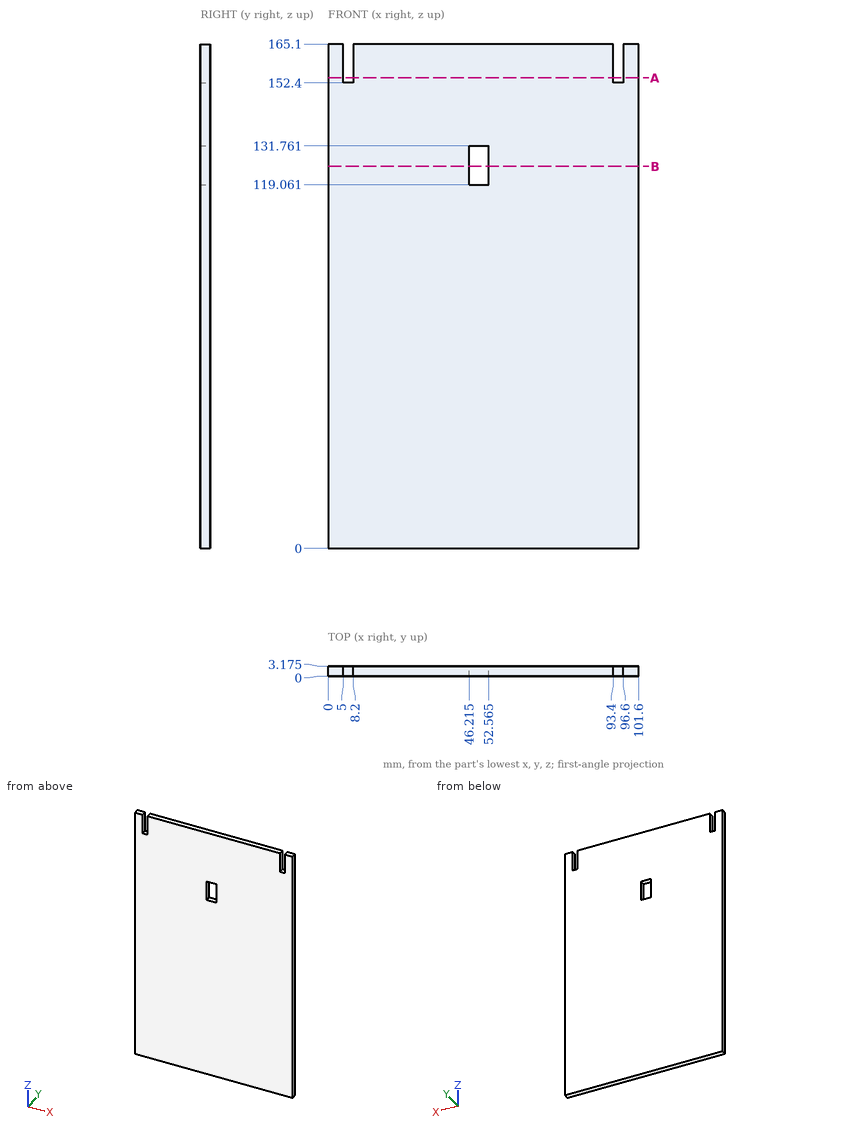
Geometry check sheet. Reference: drawing and pictorial views, mm from the part's lowest x, y, z. Give positions to 0.01 mm unless a question says otherwise; leave off trailing zeros. Loops run counter-clockwise (first coordinate to the right, second up) from the corner with the lowest first, then second, coordinate; pieces in that order, holes last. Notation, with made-up numbers: (-8.5, 63.5) - (34.5, 63.5) arc R29 ccw to (34.5, 102.5) - close; hole circle Ø6 at (65, -38.75). An arc over 180 degrees is marked (long way). Use CSV: the item, a comma, the result in double quotes. Start each with the question number.
Q1. Section check B-B, the plane z = 125. Record the cut outline in (x, y) (1 decimal).
Q2. Go/stop test with a flat-tipped pin: pin 1 Ø1.6 at (x, y) = (6.5, 1.5) entering from +Z. Record where the tip stops, or that it passes through.
Q3. Scan lines: probe 1 along X at (y, z) = (2.55, 127) (1 decimal); probe 2 along Z at (x, y) = (46.5, 1.8); probe 3 along Z at (x, y) = (95.5, 1.6). Record each from-to range of solid material in increasing order. Write a range as from..to.
Q4. Section check A-A, the plane z = 154. Record the cut outline in (x, y) (1 decimal).
Findings below:
1,outline,"(0, 0) - (46.2, 0) - (46.2, 3.2) - (0, 3.2) - close; (52.6, 0) - (101.6, 0) - (101.6, 3.2) - (52.6, 3.2) - close"
2,pin 1,"stops at z = 152.4"
3,probe 1,"x = 0..46.2, 52.6..101.6"
3,probe 2,"z = 0..119.06, 131.76..165.1"
3,probe 3,"z = 0..152.4"
4,outline,"(0, 0) - (5, 0) - (5, 3.2) - (0, 3.2) - close; (8.2, 0) - (93.4, 0) - (93.4, 3.2) - (8.2, 3.2) - close; (96.6, 0) - (101.6, 0) - (101.6, 3.2) - (96.6, 3.2) - close"
